The model under review builds one solid part; all positions refer to its coordinate system, in mm. Face numbers are marked on the shaded views. A direction names the side the tool comes from. Round coordinates to 2 decimals unless told otherwise and drop trailing zeros. Order: outer loops, then holes, each group sorted by start corner. A loop starts at its lowest first (then second) coordinate and runs counter-clockwise, first axis right, second up. Notation, with made-up numbers: (-3, 77) -> (56, 77) arc R10 ccw to (56, 88) -> close; hole circle Ø1 at (2.5, 24). An arc over 180 degrees is marked (long way). Use a Markdown table: item, result. Add a question column.
```python
from build123d import *

# Parameters (mm, degrees)
BOSS_EXTRUDE2_DEPTH = 8
FILLET1_R           = 10
FILLET3_R           = 5
FILLET4_R           = 5
SKETCH3_R           = 5
BOSS_EXTRUDE3_DEPTH = 10
SKETCH2_R           = 5
BOSS_EXTRUDE4_DEPTH = 18
SKETCH4_R           = 7
BOSS_EXTRUDE5_DEPTH = 31.6
CUT_EXTRUDE1_START  = -8
CUT_EXTRUDE1_DEPTH  = 8
SKETCH7_W           = 0.7
SKETCH7_H           = 1.2
CIRPATTERN1_COUNT   = 3
SKETCH8_R           = 3.4
CUT_EXTRUDE2_DEPTH  = 14


with BuildPart() as part:
    # Sketch1 → Boss-Extrude2 (new body)
    with BuildSketch(Plane.YZ):
        with BuildLine():
            Line((-19.991801075, -0.572616617), (-46.319219382, -15.772758664))
            Line((-46.319219382, -15.772758664), (-36.819219382, -32.227241336))
            Line((-36.819219382, -32.227241336), (-10.491801075, -17.027099289))
            ThreePointArc((-10.491801075, -17.027099289), (0, -20), (10.491801075, -17.027099289))
            Line((10.491801075, -17.027099289), (36.819219382, -32.227241336))
            Line((36.819219382, -32.227241336), (46.319219382, -15.772758664))
            Line((46.319219382, -15.772758664), (19.991801075, -0.572616617))
            ThreePointArc((19.991801075, -0.572616617), (17.320508076, 10), (9.5, 17.599715907))
            Line((9.5, 17.599715907), (9.5, 48))
            Line((9.5, 48), (-9.5, 48))
            Line((-9.5, 48), (-9.5, 17.599715907))
            ThreePointArc((-9.5, 17.599715907), (-17.320508076, 10), (-19.991801075, -0.572616617))
        make_face()
    extrude(amount=BOSS_EXTRUDE2_DEPTH)

    # Fillet1
    fillet1_edges = [part.edges().sort_by_distance(p)[0] for p in [
        (4, 9.5, 17.599715907),
        (4, 19.991801075, -0.572616617),
        (4, 10.491801075, -17.027099289),
        (4, -10.491801075, -17.027099289),
        (4, -19.991801075, -0.572616617),
        (4, -9.5, 17.599715907),
    ]]
    fillet(fillet1_edges, radius=FILLET1_R)

    # Fillet3
    fillet3_edges = [part.edges().sort_by_distance(p)[0] for p in [
        (4, -9.5, 48),
        (4, 9.5, 48),
    ]]
    fillet(fillet3_edges, radius=FILLET3_R)

    # Fillet4
    fillet4_edges = [part.edges().sort_by_distance(p)[0] for p in [
        (4, 46.319219382, -15.772758664),
        (4, 36.819219382, -32.227241336),
        (4, -36.819219382, -32.227241336),
        (4, -46.319219382, -15.772758664),
    ]]
    fillet(fillet4_edges, radius=FILLET4_R)

    # Sketch3 → Boss-Extrude3 (add)
    with BuildSketch(Plane(origin=(0, 0, 0), x_dir=(0, -1, 0), z_dir=(-1, 0, 0))):
        with Locations(Location((0, 0, 0), (0, 0, 270))):
            Circle(SKETCH3_R)
    extrude(amount=BOSS_EXTRUDE3_DEPTH)

    # Sketch2 → Boss-Extrude4 (add)
    with BuildSketch(Plane(origin=(0, 0, 0), x_dir=(0, -1, 0), z_dir=(-1, 0, 0))):
        with Locations(Location((0, 42, 0), (0, 0, 270))):
            Circle(SKETCH2_R)
        with Locations(Location((-36.373066959, -21, 0), (0, 0, 270))):
            Circle(SKETCH2_R)
        with Locations(Location((36.373066959, -21, 0), (0, 0, 270))):
            Circle(SKETCH2_R)
    extrude(amount=BOSS_EXTRUDE4_DEPTH)

    # Sketch4 → Boss-Extrude5 (add)
    with BuildSketch(Plane.YZ.offset(8)):
        with Locations(Location((0, 0, 0), (0, 0, 270))):
            Circle(SKETCH4_R)
    extrude(amount=BOSS_EXTRUDE5_DEPTH)

    # Sketch5 → Cut-Extrude1 (cut)
    with BuildSketch(Plane.YZ.offset(39.6).offset(CUT_EXTRUDE1_START)):
        with BuildLine():
            Line((-4.45, -5.403471107), (4.45, -5.403471107))
            ThreePointArc((4.45, -5.403471107), (0, -7), (-4.45, -5.403471107))
        make_face()
    extrude(amount=CUT_EXTRUDE1_DEPTH, mode=Mode.SUBTRACT)

    # Sketch7 → Cut-Revolve1 (revolve, cut)
    with BuildSketch(Plane(origin=(0, 0, 0), x_dir=(-1, 0, 0), z_dir=(0, 1, 0))):
        with Locations((8.35, 47)):
            Rectangle(SKETCH7_W, SKETCH7_H)
        with Locations((17.05, 47)):
            Rectangle(SKETCH7_W, SKETCH7_H)
    cut_revolve1 = revolve(axis=Axis((-21.815535784, 0, 42), (1, 0, 0)), mode=Mode.SUBTRACT)

    # CirPattern1: Cut-Revolve1 ×3 about axis
    cirpattern1_axis = Axis((0, 0, 0), (1, 0, 0))
    for i in range(1, CIRPATTERN1_COUNT):
        add(cut_revolve1.rotate(cirpattern1_axis, i * 360 / CIRPATTERN1_COUNT), mode=Mode.SUBTRACT)

    # Sketch8 → Cut-Extrude2 (cut)
    with BuildSketch(Plane.YZ.offset(39.6)):
        with Locations(Location((0, 0, 0), (0, 0, 270))):
            Circle(SKETCH8_R)
    extrude(amount=-CUT_EXTRUDE2_DEPTH, mode=Mode.SUBTRACT)


solid = part.part
```
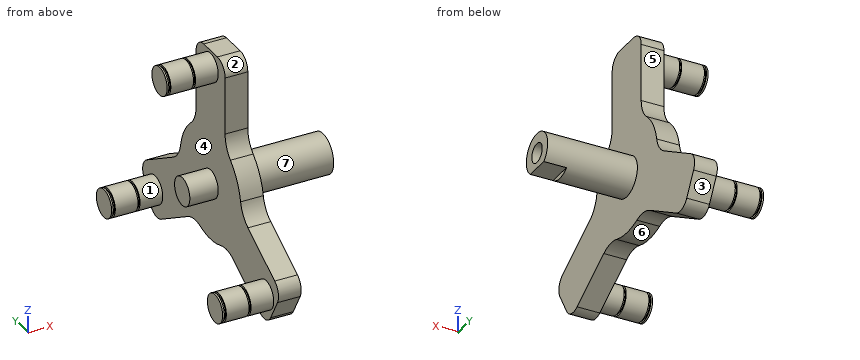
Q1. Wall thickness on line 1 (Y direction, x = 33, z = 0); line 2 (X direction, y = -9.5, z = 19.5); line 3 (Y direction, x = 33, z = 3): over which ranges is each line inside the solid? List them lowest first. Write a range as [from, to].
Q2. Add section C-C (x = 36). Write out the cut boundary in (y, z).
Q3. Add section B-B (z = 0). Write out the cut boundary in (x, y), then the cut area to 3 significant figures.
Q4. Mouldability with a two-part tool opening along Y and no side actions: class the marked faces 1, 2 and 3 as pulls with the +Y half, pulls with the -Y half, needs draft (parallel to the pull), parting line crosses it, or undercut.
Q5. Add section A-A (x = 1.5). Write out the cut boundary in (y, z), then the cut area to 3 significant figures.
Q6. Insertion check: pin 1 (8 mm diameter, centred on y = 36, z = -23.5, fed in from +X); pin 2 (6.5 mm diameter, centred on x = 2.5, z = 31, fed in from -Y); pin 3 (8 mm diameter, centred on y = 1, z = -2.5, fed in from -X). Each pin has a flat end and moves straight along its axis. Give the tip position at first contact, or say it passes through.
Q7. Add section D-D (z = 26.5). Write out the cut boundary in (x, y).
Q8. Machinability: for the marked faces 4, 5, 6 and 7, which of the approach directions +Z, -Z, +X, -X, +Y, -Y give a long, thin tool a straight path to every point of the face, cutting with its end or side? Answer none if there is none.
Report:
| question | item | result |
|---|---|---|
| 1 | line 1 | y = [-7, -3.4], [3.4, 7] |
| 1 | line 2 | x = [0, 8] |
| 1 | line 3 | y = [-6.32, -1.6], [1.6, 6.32] |
| 2 | outline | (-4.45, -5.4) -> (4.45, -5.4) arc R7 ccw (long way) to start; hole circle Ø6.8 at (0, 0) |
| 3 | outline | (-10, -5) -> (0, -5) -> (0, -21.13) -> (8, -21.13) -> (8, -7) -> (39.6, -7) -> (39.6, -3.4) -> (25.6, -3.4) -> (25.6, 3.4) -> (39.6, 3.4) -> (39.6, 7) -> (8, 7) -> (8, 21.13) -> (0, 21.13) -> (0, 5) -> (-10, 5) -> close |
| 3 | area | 785 mm² |
| 4 | face 1 | undercut |
| 4 | face 2 | pulls with the -Y half |
| 4 | face 3 | pulls with the +Y half |
| 5 | outline | (-43.82, -20.1) -> (-39.32, -27.9) arc R5 ccw to (-32.49, -29.73) -> (-14.99, -19.63) arc R10 cw to (-6.66, -18.86) arc R20 ccw to (6.66, -18.86) arc R10 cw to (14.99, -19.63) -> (32.49, -29.73) arc R5 ccw to (39.32, -27.9) -> (43.82, -20.1) arc R5 ccw to (41.99, -13.27) -> (24.49, -3.17) arc R10 cw to (19.66, 3.66) arc R20 ccw to (13, 15.2) arc R10 cw to (9.5, 22.8) -> (9.5, 43) arc R5 ccw to (4.5, 48) -> (-4.5, 48) arc R5 ccw to (-9.5, 43) -> (-9.5, 22.8) arc R10 cw to (-13, 15.2) arc R20 ccw to (-19.66, 3.66) arc R10 cw to (-24.49, -3.17) -> (-41.99, -13.27) arc R5 ccw to start |
| 5 | area | 2,890 mm² |
| 6 | pin 1 | stops at x = 8 |
| 6 | pin 2 | stops at y = -9.5 |
| 6 | pin 3 | stops at x = -10 |
| 7 | outline | (0, -9.5) -> (8, -9.5) -> (8, 9.5) -> (0, 9.5) -> close |
| 8 | face 4 | -X |
| 8 | face 5 | +Z, +X, -X, +Y |
| 8 | face 6 | -Z, +X, -X |
| 8 | face 7 | +X |
